Autodesk Inventor part; units mm, degrees
ref_plane "XZ Plane" through (0, 0, 0) normal (0, 1, 0) x (-1, 0, 0)
ref_plane "XY Plane" through (0, 0, 0) normal (0, 0, 1) x (1, 0, 0)
sketch "Sketch1" plane through (0, 0, 0) normal (0, 0, 1) x (1, 0, 0)
  circle A0 centre (-7.65, 0) radius 1.25
  line L0 (0, 4.1624) -> (0, -4.1624)
  point P0 (0, 0)
  dimension "d0" = 2.5
revolve "Revolution1" add sketch "Sketch1" angle 360 about axis through (0, 4.1624, 0) along (0, -1, 0)
ref_plane "Work Plane1" through (21.6, 0, 0) normal (1, 0, 0) x (0, 1, 0)
sketch "Sketch2" plane through (21.6, 0, 0) normal (1, 0, 0) x (0, 1, 0)
  circle A0 centre (0, 0) radius 1.5
  circle A1 centre (0, 0) radius 2.5
  dimension "d3" = 3
  dimension "d4" = 5
ref_plane "Work Plane2" through (8.9, 0, 0) normal (1, 0, 0) x (0, 1, 0)
sketch "Sketch3" plane through (8.9, 0, 0) normal (1, 0, 0) x (0, 1, 0)
  circle A0 centre (0, 0) radius 3.5297
  circle A1 centre (0, 0) radius 1.487
extrude "Extrusion1" add sketch "Sketch3" along normal blind 2.54
extrude "Extrusion2" add sketch "Sketch2" against normal blind 2.54
sketch "Sketch5" plane through (11.44, 0, 0) normal (1, 0, 0) x (0, 0, -1)
  circle A0 centre (0, 0) radius 1.5
  circle A1 centre (0, 0) radius 2.9723
sketch "Sketch6" plane through (19.06, 0, 0) normal (-1, 0, 0) x (0, 0, 1)
  circle A0 centre (0, 0) radius 2.5
  circle A1 centre (0, 0) radius 1.5
  circle A2 centre (0, 0) radius 2.5
sketch "Sketch7" plane through (0, 0, 0) normal (0, 1, 0) x (-1, 0, 0)
  point P0 (0, 0)
extrude "Extrusion3" add sketch "Sketch5" along normal blind 2.54
sketch "Sketch8" plane through (13.98, 0, 0) normal (1, 0, 0) x (0, 0, -1)
  circle A0 centre (0, 0) radius 1.487
  circle A1 centre (0, 0) radius 2.7524
extrude "Extrusion4" add sketch "Sketch8" along normal blind 5.588
sketch "Sketch9" plane through (8.9, 0, 0) normal (1, 0, 0) x (0, 1, 0)
  circle A0 centre (0, 0) radius 3.5297
ref_plane "Work Plane3" through (6.36, 0, 0) normal (1, 0, 0) x (0, 1, 0)
sketch "Sketch10" plane through (6.36, 0, 0) normal (1, 0, 0) x (0, 1, 0)
  circle A0 centre (0, 0) radius 1.578
loft "Loft1" add profiles "Sketch10" section 2 edges at (8.9, -3.5297, 0)
sketch "Sketch11" plane through (21.6, 0, 0) normal (1, 0, 0) x (0, 1, 0)
  circle A0 centre (0, 0) radius 1.5635
extrude "Extrusion5" cut sketch "Sketch11" against normal blind 12.7
sketch "Sketch12" plane through (21.6, 0, 0) normal (1, 0, 0) x (0, 1, 0)
  circle A0 centre (0, 0) radius 1.5635
  circle A1 centre (0, 0) radius 3.9487
extrude "Extrusion6" cut sketch "Sketch12" against normal blind 4.318
properties part number "kims_perch2020"
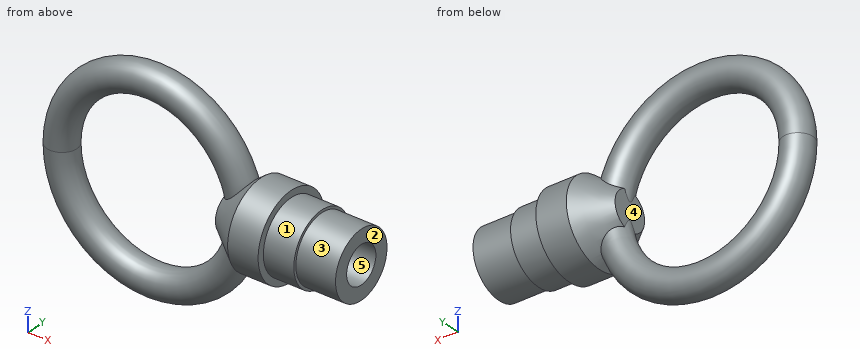
The model under review builds one solid part; all positions refer to its coordinate system, in mm. Face numbers are marked on the shaded views. A direction names the side the tool comes from. Give positions to 0.01 mm unless a question says otherwise; leave off trailing zeros. Loops run counter-clockwise (first coordinate to the right, second up) from the corner with the lowest first, then second, coordinate; pieces in that order, holes last. Notation, with made-up numbers: (36, -12.75) - (45, -12.75) arc R11 cw to (45, 7.25) - close; hole circle Ø4 at (75.25, 78.25). An arc over 180 degrees is marked (long way). Answer as a JSON object with one key per item and string values.
Q1. For the marked faces 1 and 2, list the 3-axis set-ups (+Z, -Z, +X, -X, +Y, -Y) from which the entire face can be reached by the end or side of a thin tool; tool diameter is ignored.
Worked out:
{"face 1": "+X", "face 2": "+Z, -Z, +X, +Y, -Y"}
Q2. To check wall thickness, follow line 1 along Z through (x, y) = (15, 0); line 2 along X through (y, z) = (1.5, 0); line 3 along X through (y, z) = (0, -4.75). State the ranges of each line that lie inside material, in increasing order.
Worked out:
{"line 1": "z = -2.75 to -1.56, 1.56 to 2.75", "line 2": "x = 6.36 to 8.9", "line 3": "x = -7.53 to -4.29, 4.29 to 7.53"}
Q3. Mouldability with a two-part tool opening along Y and no side actions: class the marked faces 3, 4 and 5 as +Y half, -Y half, draft (parallel to the pull), parting line (faces both ways), or undercut.
Worked out:
{"face 3": "parting line", "face 4": "draft", "face 5": "undercut"}
Q4. Add section A-A on y = 0. State the section outline as (x, z) points.
Worked out:
{"outline": "(8.34, -3.1) - (8.9, -3.53) - (11.44, -3.53) - (11.44, -2.97) - (13.98, -2.97) - (13.98, -2.75) - (17.28, -2.75) - (17.28, -1.56) - (8.9, -1.56) - (8.9, 1.56) - (17.28, 1.56) - (17.28, 2.75) - (13.98, 2.75) - (13.98, 2.97) - (11.44, 2.97) - (11.44, 3.53) - (8.9, 3.53) - (8.34, 3.1) arc R8.9 ccw (long way) to start; hole (6.36, -0.71) - (6.36, 0.71) arc R6.4 ccw (long way) to start"}
Q5. Insertion check: pin 1 (1.5 mm diameter, centred on x = 9.5, y = 2.5, fed in from +Z); pin 2 (2 mm diameter, centred on x = 13, z = 5, fed in from +Y); pin 3 (2 mm diameter, centred on x = 2.5, y = 1, fed in from +Z); pin 4 (2 mm diameter, centred on x = 4.5, z = -4.5, fed in from -Y). Each pin has a flat end and moves straight along its axis. Give the tip position at first contact, or say it passes through.
Worked out:
{"pin 1": "stops at z = 3.07", "pin 2": "passes through", "pin 3": "stops at z = 8.68", "pin 4": "stops at y = -1.22"}
